Source: CAD feature listing. Evaluate the final solid. Frame: model axes, mm. Round coordinates to 2 decimals unless told otherwise and drop trailing zeros. Answer as a JSON object with one key per item and string values.
from build123d import *

# Parameters (mm, degrees)
SKETCH_28_R               = 2.075
EXTRUDE_2020V_DEPTH       = 240
HOLE_WIZARD_1_2020V_D     = 4.2
HOLE_WIZARD_1_2020V_DEPTH = 12.4
HOLE_WIZARD_1_2020V_TIP   = 1.2618073
HOLE_WIZARD_2_2020V_D     = 4.2
HOLE_WIZARD_2_2020V_DEPTH = 12.4
HOLE_WIZARD_2_2020V_TIP   = 1.2618073


with BuildPart() as part:
    # 草图28 → 2020V (new body)
    with BuildSketch(Plane(origin=(0, 0, 0), x_dir=(1, 0, 0), z_dir=(0, 1, 0))):
        with BuildLine():
            Line((-3.900000395, 2.839340223), (-3.900000395, 0.282843107))
            Line((-3.900000395, 0.282843107), (-3.617157288, 0))
            Line((-3.617157288, 0), (-3.9, -0.282842712))
            Line((-3.9, -0.282842712), (-3.9, -2.839339828))
            Line((-3.9, -2.839339828), (-6.560660172, -5.5))
            Line((-6.560660172, -5.5), (-8.2, -5.5))
            Line((-8.2, -5.5), (-8.2, -3.150000255))
            Line((-8.2, -3.150000255), (-10, -4.950000255))
            Line((-10, -4.950000255), (-10, -9.5))
            ThreePointArc((-10, -9.5), (-9.853553391, -9.853553391), (-9.5, -10))
            Line((-9.5, -10), (-4.950000255, -10))
            Line((-4.950000255, -10), (-3.150000255, -8.2))
            Line((-3.150000255, -8.2), (-5.5, -8.2))
            Line((-5.5, -8.2), (-5.5, -6.560660172))
            Line((-5.5, -6.560660172), (-2.839339828, -3.9))
            Line((-2.839339828, -3.9), (-0.282842712, -3.9))
            Line((-0.282842712, -3.9), (0, -3.617157288))
            Line((0, -3.617157288), (0.282842712, -3.9))
            Line((0.282842712, -3.9), (2.839339828, -3.9))
            Line((2.839339828, -3.9), (5.5, -6.560660172))
            Line((5.5, -6.560660172), (5.5, -8.2))
            Line((5.5, -8.2), (3.150000255, -8.2))
            Line((3.150000255, -8.2), (4.950000255, -10))
            Line((4.950000255, -10), (9.5, -10))
            ThreePointArc((9.5, -10), (9.853553391, -9.853553391), (10, -9.5))
            Line((10, -9.5), (10, -4.950000255))
            Line((10, -4.950000255), (8.2, -3.150000255))
            Line((8.2, -3.150000255), (8.2, -5.5))
            Line((8.2, -5.5), (6.560660172, -5.5))
            Line((6.560660172, -5.5), (3.9, -2.839339828))
            Line((3.9, -2.839339828), (3.9, -0.282842712))
            Line((3.9, -0.282842712), (3.617157288, 0))
            Line((3.617157288, 0), (3.900000116, 0.282842829))
            Line((3.900000116, 0.282842829), (3.900000116, 2.839339944))
            Line((3.900000116, 2.839339944), (6.560660288, 5.500000116))
            Line((6.560660288, 5.500000116), (8.200000116, 5.500000116))
            Line((8.200000116, 5.500000116), (8.200000116, 3.150000371))
            Line((8.200000116, 3.150000371), (10.000000116, 4.950000371))
            Line((10.000000116, 4.950000371), (10.000000116, 9.499999884))
            ThreePointArc((10.000000116, 9.499999884), (9.853553507, 9.853553275), (9.500000116, 9.999999884))
            Line((9.500000116, 9.999999884), (4.950000139, 9.999999884))
            Line((4.950000139, 9.999999884), (3.150000139, 8.199999884))
            Line((3.150000139, 8.199999884), (5.499999884, 8.199999884))
            Line((5.499999884, 8.199999884), (5.499999884, 6.560660056))
            Line((5.499999884, 6.560660056), (2.839339712, 3.899999884))
            Line((2.839339712, 3.899999884), (0.282842991, 3.899999884))
            Line((0.282842991, 3.899999884), (0, 3.617156893))
            Line((0, 3.617156893), (-0.282842712, 3.899999605))
            Line((-0.282842712, 3.899999605), (-2.839339434, 3.899999605))
            Line((-2.839339434, 3.899999605), (-5.499999605, 6.560659777))
            Line((-5.499999605, 6.560659777), (-5.499999605, 8.199999605))
            Line((-5.499999605, 8.199999605), (-3.149999861, 8.199999605))
            Line((-3.149999861, 8.199999605), (-4.949999861, 9.999999605))
            Line((-4.949999861, 9.999999605), (-9.500000395, 9.999999605))
            ThreePointArc((-9.500000395, 9.999999605), (-9.853553785, 9.853552996), (-10.000000395, 9.499999605))
            Line((-10.000000395, 9.499999605), (-10.000000395, 4.95000065))
            Line((-10.000000395, 4.95000065), (-8.200000395, 3.15000065))
            Line((-8.200000395, 3.15000065), (-8.200000395, 5.500000395))
            Line((-8.200000395, 5.500000395), (-6.560660566, 5.500000395))
            Line((-6.560660566, 5.500000395), (-3.900000395, 2.839340223))
        make_face()
        with Locations(Location((0, 0, 0), (0, 0, 270))):
            Circle(SKETCH_28_R, mode=Mode.SUBTRACT)
    extrude(amount=EXTRUDE_2020V_DEPTH)

    # 1-2020V
    with Locations(Plane(origin=(0, 240, 0), x_dir=(1, 0, 0), z_dir=(0, 1, 0))):
        with Locations((0, 0)):
            Hole(HOLE_WIZARD_1_2020V_D / 2, depth=HOLE_WIZARD_1_2020V_DEPTH)
            with Locations((0, 0, -(HOLE_WIZARD_1_2020V_DEPTH + HOLE_WIZARD_1_2020V_TIP / 2))):  # 118° drill point
                Cone(0, HOLE_WIZARD_1_2020V_D / 2, HOLE_WIZARD_1_2020V_TIP, mode=Mode.SUBTRACT)

    # 2-2020V
    with Locations(Plane(origin=(0, 0, 0), x_dir=(-1, 0, 0), z_dir=(0, -1, 0))):
        with Locations((0, 0)):
            Hole(HOLE_WIZARD_2_2020V_D / 2, depth=HOLE_WIZARD_2_2020V_DEPTH)
            with Locations((0, 0, -(HOLE_WIZARD_2_2020V_DEPTH + HOLE_WIZARD_2_2020V_TIP / 2))):  # 118° drill point
                Cone(0, HOLE_WIZARD_2_2020V_D / 2, HOLE_WIZARD_2_2020V_TIP, mode=Mode.SUBTRACT)


solid = part.part
Item 1: Pull-direction query (X, two-part tool) for faces 1 (the flat face through (10, 118, -7)), 2 (the flat face through (7, 118, -10)), 3 (the cylindrical face through (-2.003, 233.713, -0.631)); classes: pulls with the +X half, pulls with the -X half, needs draft (parallel to the pull), parting line crosses it, or undercut.
Answer sheet:
{"face 1": "pulls with the +X half", "face 2": "needs draft", "face 3": "undercut"}
Item 2: Line query: probe 1 along X at (y, z) = (186, -5); probe 2 along X at (y, z) = (110.5, 0) (3 decimals); probe 3 along X at (y, z) = (190, -4.5). Output: solid intervals per line, ascending. Write a range as from..to.
Answer sheet:
{"probe 1": "x = -10..-8.2, -6.06..-3.94, 3.94..6.06, 8.2..10", "probe 2": "x = -3.617..-2.075, 2.075..3.617", "probe 3": "x = -9.55..-8.2, -5.56..-3.44, 3.44..5.56, 8.2..9.55"}
Item 3: Contact query for flat-ended pins moving along their axis: pin 1 Ø1 at (x, y) = (-4, 89) entering from +Z; pin 2 Ø3 at (y, z) = (99.5, -0.5) entering from -X; pin 3 Ø1.2 at (y, z) = (134, 4) entering from -X. Output: stop coordinate, or through.
Answer sheet:
{"pin 1": "stops at z = 9.55", "pin 2": "stops at x = -3.9", "pin 3": "stops at x = -9.65"}
